Autodesk Inventor part; units mm, degrees
ref_plane "YZ Plane" through (0, 0, 0) normal (1, 0, 0) x (0, 1, 0)
ref_plane "XZ Plane" through (0, 0, 0) normal (0, 1, 0) x (-1, 0, 0)
ref_plane "XY Plane" through (0, 0, 0) normal (0, 0, 1) x (1, 0, 0)
ref_plane "Work Plane1" through (0, 0, 0) normal (0, 0, 1) x (1, 0, 0)
sketch "Sketch1" plane through (0, 0, 0) normal (0, 1, 0) x (-1, 0, 0)
  line L0 (-11.125, -7) -> (11.125, -7)
  line L1 (11.125, -7) -> (11.125, 0)
  line L2 (11.125, 0) -> (-11.125, 0)
  line L3 (-11.125, 0) -> (-11.125, -7)
  line L4 (-11.125, -7) -> (11.125, 0) construction
  line L5 (11.125, -7) -> (-11.125, 0) construction
  line L6 (0, -3.5) -> (0, 0) construction
  line L7 (-11.125, 0) -> (-15.55, 0)
  line L8 (-15.55, 0) -> (-12.125, -3.425)
  line L9 (-12.125, -3.575) -> (-15.55, -7)
  line L10 (-15.55, -7) -> (-11.125, -7) construction
  line L11 (-12.125, -3.425) -> (-12.125, -3.575)
  line L12 (-15.55, -7) -> (-14.8221, -9)
  line L13 (-14.8221, -9) -> (-10.2279, -9)
  line L14 (-10.2279, -9) -> (-9.5, -7)
  dimension "d0" = 22.25
  dimension "d1" = 7
  dimension "d3" = 45
  dimension "d4" = 45
  dimension "d6" = 70
  dimension "d7" = 2
  dimension "d8" = 19
  dimension "d9" = 70
  dimension "d16" = 1
  dimension "d17" = 31.1
revolve "Revolution1" add sketch "Sketch1" angle 360 about axis through (0, 0, -3.5) along (0, 0, 1) contours L0 L14 L13 L12 L9 L11 L8 L7 L3
fillet "Fillet1" radius 0.6 4 edges at (-15.55, 0, 0) (-15.55, 0, -7) (-14.8221, 0, -9) (-10.2279, 0, -9)
chamfer "Chamfer1" distance 0.6 angle 45 1 edges at (-11.125, 0, 0)
properties part number "vroller_3DPrint"
Source: CAD feature listing. Evaluate the final solid. Frame: model axes, mm. A direction names the side the tool comes from. Coordinates: 2 decimals unless noted, no trailing zeros. Loops run counter-clockwise (first coordinate to the right, second up) from the corner with the lowest first, then second, coordinate; pieces in that order, holes last. Notation, with made-up numbers: (-37, -1) - (-26, -1) arc R28 cw to (-26, 28) - close; hole circle Ø7 at (79.5, 63). An arc over 180 degrees is marked (long way). One line per item, written item: value. Start each with the question number.
1. Section A-A (z = -5.5). Return the cut outline in (x, y) (3 decimals).
2. Contact query for flat-ended pins moving along their axis: P1, Ø1.5, axis at y = 3, z = -3.5, coming from the +X side; P2, Ø2, axis at y = 7.5, z = -1.5, coming from the +X side; P3, Ø11, axis at x = -3.5, y = 2.5, coming from the +Z side. Output: stop coordinate, or through.
3. Section B-B (z = -2.75). Return the cut outline in (x, y) (3 decimals).
4. Set-up query: faces 1 (the flat face through (-12, 2, 0)), 2 (the conical face through (-9.08, -8.33, -3.77)), 3 (the flat face through (-5, 8.3, -7)). Return all of +Z, -Z, +X, -X, +Y, -Y with unobstructed straight access to the full face (end or side cutting, diameter ignored); none if empty.
5. Ray query, L1, parallel to Y at x = 0, z = -3.5 (3 decimals); L2, parallel to Z at x = -5.5, y = 9.5; L3, parallel to Y at x = -7, z = -4. Return the intervals inside material, ascending.
6. Mould query, pull axis Z, two halves, no side actions, for faces 4 (the flat face through (-9, -6, -9)), 5 (the conical face through (11.71, 3.69, -3.27)), 6 (the cylindrical face through (-8.2, -7.52, -3.84)). Classes: pulls with the +Z half, pulls with the -Z half, needs draft (parallel to the pull), parting line crosses it, or undercut.
Verdict:
1. outline: circle Ø28.1 at (0, 0); hole circle Ø22.25 at (0, 0)
2. P1: stops at x = 12.46
2. P2: stops at x = 13
2. P3: stops at z = -7
3. outline: circle Ø25.6 at (0, 0); hole circle Ø22.25 at (0, 0)
4. face 1: +Z, +X, -X, +Y, -Y
4. face 2: none
4. face 3: +Z
5. L1: y = -12.125 to -11.125, 11.125 to 12.125
5. L2: z = -9 to -7
5. L3: y = -10.42 to -8.65, 8.65 to 10.42
6. face 4: pulls with the -Z half
6. face 5: undercut
6. face 6: needs draft
